Design review of the part built by this model. Coordinates are the model's own, in mm. Face numbers are marked on the shaded views. Give positions to 0.01 mm unless a question says otherwise; leave off trailing zeros. Order: outer loops, then holes, each group sorted by start corner. A loop starts at its lowest first (then second) coordinate and runs counter-clockwise, first axis right, second up. Notation, with made-up numbers: (89.25, 60.25) - (117.25, 60.25) arc R17 cw to (117.25, 93.25) - close; hole circle Ø11 at (-29.75, -23). An arc over 180 degrees is marked (long way). Write each question's results on one line, items separated by ' | '. Start each with the question number.
Autodesk Inventor part; units mm, degrees
ref_plane "YZ Plane" through (0, 0, 0) normal (1, 0, 0) x (0, 1, 0)
ref_plane "XZ Plane" through (0, 0, 0) normal (0, 1, 0) x (-1, 0, 0)
ref_plane "XY Plane" through (0, 0, 0) normal (0, 0, 1) x (1, 0, 0)
sketch "Sketch1" plane through (0, 0, 0) normal (0, 0, 1) x (1, 0, 0)
  circle A0 centre (0, 0) radius 7.25
  dimension "d0" = 14.5
extrude "Extrusion1" add sketch "Sketch1" against normal blind 5
hole "Hole1" at (0, 0, 0) direction (0, 0, -1) diameter 6.35 end through all countersink diameter 10 countersink angle 90
fillet "Fillet1" radius 0.5 2 edges at (-7.25, 0, 0) (-7.25, 0, -5)
properties part number "plate"
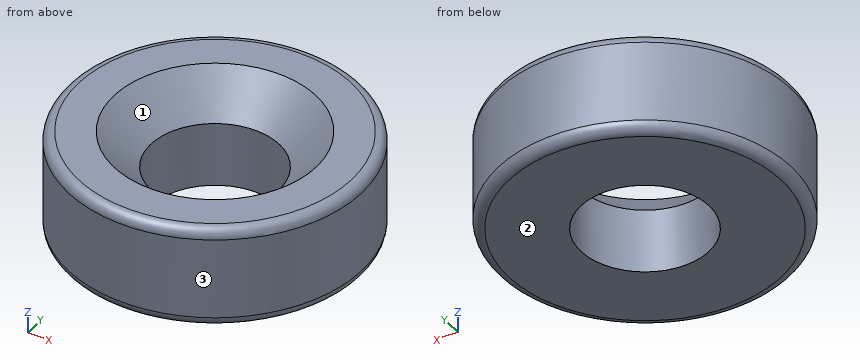
Q1. For line 1 (Y direction, x = 0, z = -3.7) (3 decimals); line 2 (X direction, y = -1, z = -1.55); line 3 (Y direction, x = 1.75, z = -1.35), list the stretches that pass through material, from the lowest coordinate up. Write a range as [from, to].
Q2. Insertion check: pin 1 Ø2 at (y, z) = (-4, -4.5) entering from +X; pin 2 Ø3 at (y, z) = (4, -3) entering from +X; pin 3 Ø1.5 at (x, y) = (1.5, -3) entering from +Z; pin 4 Ø2 at (x, y) = (5.5, 0) entering from +Z. Each pin has a flat end and moves straight along its axis. Give the tip position at first contact, or say it passes through.
Q3. Add section C-C (z = -4). Give the boundary of the cut face in (x, y) (3 decimals).
Q4. Add section A-A (x = 0). Give the boundary of the cut face in (y, z) (3 decimals).
Q5. Draft analysis for pull direction Y (two halves, no side actions). For the marked faces 1, 2 and 3, state which applies: pulls with the +Y half, pulls with the -Y half, needs draft (parallel to the pull), parting line crosses it, or undercut.
Verdict:
1) line 1: y = [-7.25, -3.175], [3.175, 7.25] | line 2: x = [-7.18, -3.3], [3.3, 7.18] | line 3: y = [-7.04, -3.2], [3.2, 7.04]
2) pin 1: stops at x = 6.6 | pin 2: stops at x = 6.81 | pin 3: stops at z = -0.9 | pin 4: stops at z = 0
3) outline: circle Ø14.5 at (0, 0); hole circle Ø6.35 at (0, 0)
4) outline: (-7.25, -4.5) arc R0.5 ccw to (-6.75, -5) - (-3.175, -5) - (-3.175, -1.825) - (-5, 0) - (-6.75, 0) arc R0.5 ccw to (-7.25, -0.5) - close; (3.175, -5) - (6.75, -5) arc R0.5 ccw to (7.25, -4.5) - (7.25, -0.5) arc R0.5 ccw to (6.75, 0) - (5, 0) - (3.175, -1.825) - close
5) face 1: undercut | face 2: needs draft | face 3: parting line crosses it
